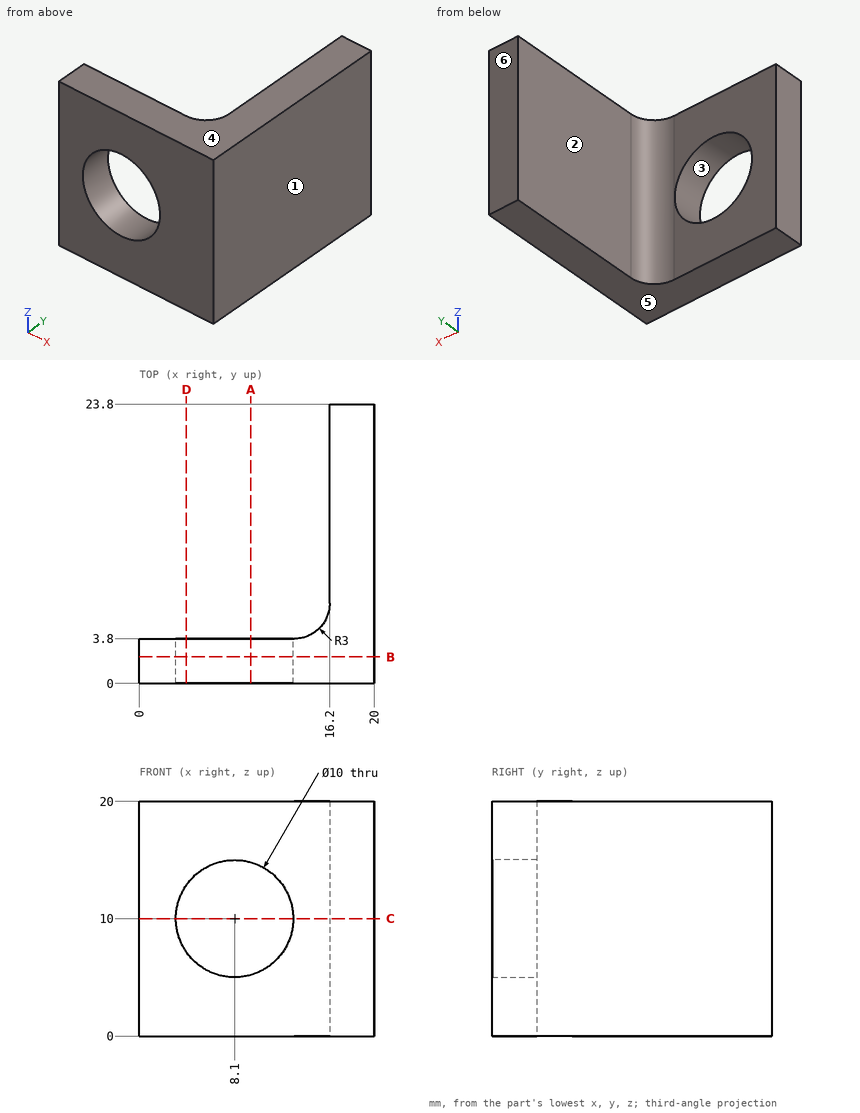
Here's the drawing with two shaded views (mm, measured from the low corner). I have some questions. A direction names the side the tool comes from. Give positions to 0.01 mm unless a question says otherwise; leave off trailing zeros. Loops run counter-clockwise (first coordinate to the right, second up) from the corner with the lowest first, then second, coordinate; pieces in that order, holes last. Notation, with made-up numbers: (86, 21.5) -> (118, 21.5) arc R10 ccw to (118, 33.5) -> close; hole circle Ø10 at (58.25, 60). An arc over 180 degrees is marked (long way). Use one line per item in the form item = value.
1) If we section it at B-B (y = 2.25): Please give me the cut outline in (x, z), plus the area to 3 significant figures.
Answers:
outline = (0, 0) -> (20, 0) -> (20, 20) -> (0, 20) -> close; hole circle Ø10 at (8.1, 10)
area = 321 mm²
2) If we section it at D-D (x = 4): Please give me the cut outline in (y, z).
Answers:
outline = (0, 0) -> (3.8, 0) -> (3.8, 7.14) -> (0, 7.14) -> close; (0, 12.86) -> (3.8, 12.86) -> (3.8, 20) -> (0, 20) -> close
3) If we section it at A-A (x = 9.5): Please give me the cut outline in (y, z), plus the area to 3 significant figures.
Answers:
outline = (0, 0) -> (3.8, 0) -> (3.8, 5.2) -> (0, 5.2) -> close; (0, 14.8) -> (3.8, 14.8) -> (3.8, 20) -> (0, 20) -> close
area = 39.5 mm²
4) We'd pull the mould along Z, two halves only. Please class the marked faces 3, 4, 5 and 6: released by +Z, released by -Z, zero draft, split by the parting line, or undercut.
Answers:
face_3 = undercut
face_4 = released by +Z
face_5 = released by -Z
face_6 = zero draft
5) If we section it at C-C (z = 10): Please give me the cut outline in (x, y).
Answers:
outline = (0, 0) -> (3.1, 0) -> (3.1, 3.8) -> (0, 3.8) -> close; (13.1, 0) -> (20, 0) -> (20, 23.8) -> (16.2, 23.8) -> (16.2, 6.8) arc R3 cw to (13.2, 3.8) -> (13.1, 3.8) -> close
6) Will these pins go through, and if not, where does the flat tip stop? pin 1 (5 mm diameter, centred on x = 9.5, z = 7, fed in from +Y); pin 2 (5 mm diameter, centred on y = 12, z = 2.5, fed in from -X).
Answers:
pin_1 = 3.8
pin_2 = 16.2
7) For the marked faces 1 and 2, which set-ups out of +Z, -Z, +X, -X, +Y, -Y let a thin tool reach every point of the face, with its end or its side?
Answers:
face_1 = +Z, -Z, +X, +Y, -Y
face_2 = +Z, -Z, -X, +Y
8) I need wall thicknesses on line 1 along X through (y, z) = (1, 10); line 2 along Y through (x, z) = (12.25, 16.25); line 3 along X through (y, z) = (9.5, 1). Which ranges of each line are inside material? Lowest first, please.
Answers:
line_1 = 0 to 3.1, 13.1 to 20
line_2 = 0 to 3.8
line_3 = 16.2 to 20
